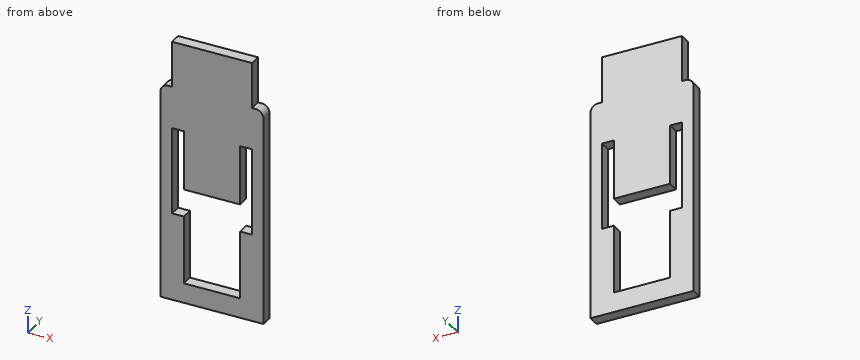
from build123d import *

# Parameters (mm, degrees)
BOSS_EXTRUDE1_DEPTH = 3
FILLET1_R           = 2


with BuildPart() as part:
    # Sketch1 → Boss-Extrude1 (new body)
    with BuildSketch(Plane(origin=(0, 0, 0), x_dir=(1, 0, 0), z_dir=(0, 1, 0))):
        Polygon((-10.45025, -22.36565), (-10.45025, -34.36565), (10.45025, -34.36565), (10.45025, -22.36565), (13.45025, -22.36565), (13.45025, 34.36565), (-13.45025, 34.36565), (-13.45025, -22.36565), align=None)
        Polygon((-7.35025, -11.36565), (-10.45025, -11.36565), (-10.45025, 11.36565), (-7.35025, 11.36565), (-7.35025, 29.16565), (7.35025, 29.16565), (7.35025, 11.36565), (10.45025, 11.36565), (10.45025, -11.36565), (7.35025, -11.36565), (7.35025, 4.16565), (-7.35025, 4.16565), align=None, mode=Mode.SUBTRACT)
    extrude(amount=BOSS_EXTRUDE1_DEPTH)

    # Fillet1
    fillet1_edges = [part.edges().sort_by_distance(p)[0] for p in [
        (-13.45025, 1.5, 22.36565),
        (13.45025, 1.5, 22.36565),
    ]]
    fillet(fillet1_edges, radius=FILLET1_R)


solid = part.part
Read the model definition and answer for the solid it produces. Units are mm, in the model's axes. Coordinates: 2 decimals unless noted, no trailing zeros. Write each loop counter-clockwise with the first axis right and the second up, starting at its lowest first coordinate (ties: lowest second). Pieces come first, ordered by that corner, then holes. Notation, with made-up numbers: M 44,69.25 L 81,69.25 A16 cw 81,83.25 Z; hole C 35.25,-35.75 d11. An arc over 180 degrees is marked long. Use a Markdown table: item, result.
Q1. The part is cut by section D-D, the plane y = 1.3. Write down the section's boundary in (x, z), then the cut area to 3 significant figures.
Answer block:
| item | result |
|---|---|
| outline | M -13.45,-34.37 L 13.45,-34.37 L 13.45,20.37 A2 ccw 11.45,22.37 L 10.45,22.37 L 10.45,34.37 L -10.45,34.37 L -10.45,22.37 L -11.45,22.37 A2 ccw -13.45,20.37 Z; hole M -10.45,-11.37 L -7.35,-11.37 L -7.35,-29.17 L 7.35,-29.17 L 7.35,-11.37 L 10.45,-11.37 L 10.45,11.37 L 7.35,11.37 L 7.35,-4.17 L -7.35,-4.17 L -7.35,11.37 L -10.45,11.37 Z |
| area | 1,270 mm2 |
Q2. The part is cut by section C-C, the plane z = -9. Write down the section's boundary in (x, y), then the cut area to 3 significant figures.
Answer block:
| item | result |
|---|---|
| outline | M -13.45,0 L -10.45,0 L -10.45,3 L -13.45,3 Z; M 10.45,0 L 13.45,0 L 13.45,3 L 10.45,3 Z |
| area | 18.0 mm2 |
Q3. The part is cut by section A-A, the plane x = 9.75. Write down the section's boundary in (y, z).
Answer block:
| item | result |
|---|---|
| outline | M 0,-34.37 L 3,-34.37 L 3,-11.37 L 0,-11.37 Z; M 0,11.37 L 3,11.37 L 3,34.37 L 0,34.37 Z |
Q4. Each of these flat-tipped pins is pushed along its axis until it touches: pin 1 Ø1.5 at (y, z) = (1.5, 28.5) entering from -X; pin 2 Ø1.5 at (y, z) = (2, 29) entering from +X. Where does it stop, or does it pass through?
Answer block:
| item | result |
|---|---|
| pin 1 | stops at x = -10.45 |
| pin 2 | stops at x = 10.45 |
Q5. The part is cut by section B-B, the plane z = 10. Write down the section's boundary in (x, y).
Answer block:
| item | result |
|---|---|
| outline | M -13.45,0 L -10.45,0 L -10.45,3 L -13.45,3 Z; M -7.35,0 L 7.35,0 L 7.35,3 L -7.35,3 Z; M 10.45,0 L 13.45,0 L 13.45,3 L 10.45,3 Z |
Q6. Straight lines are drawn through the part: L1, parallel to X at y = 0.7, z = -3; L2, parallel to Z at x = 0.75, y = 2.5; L3, parallel to Z at x = -10.25, y = 2.75. For each, find the intervals that lie inside material, in ascending order. Write a range as [from, to].
Answer block:
| item | result |
|---|---|
| L1 | x = [-13.45, -10.45], [-7.35, 7.35], [10.45, 13.45] |
| L2 | z = [-34.37, -29.17], [-4.17, 34.37] |
| L3 | z = [-34.37, -11.37], [11.37, 34.37] |
